from build123d import *

# Parameters (mm, degrees)
SKETCH2_R           = 12
BOSS_EXTRUDE1_DEPTH = 10.23
SKETCH3_R           = 2.5
CUT_EXTRUDE1_DEPTH  = 20.815471228
CHAMFER1_SIZE       = 2
CHAMFER2_SIZE       = 2


with BuildPart() as part:
    # Sketch2 → Boss-Extrude1 (new body)
    with BuildSketch(Plane.XY):
        Circle(SKETCH2_R)
    extrude(amount=BOSS_EXTRUDE1_DEPTH)

    # Sketch3 → Cut-Extrude1 (cut, through all)
    with BuildSketch(Plane.XY.offset(10.23)):
        Circle(SKETCH3_R)
    extrude(amount=-CUT_EXTRUDE1_DEPTH, mode=Mode.SUBTRACT)

    # Chamfer1
    chamfer1_edges = [part.edges().sort_by_distance(p)[0] for p in [
        (-12, 0, 10.23),
    ]]
    chamfer(chamfer1_edges, length=CHAMFER1_SIZE)

    # Chamfer2
    chamfer2_edges = [part.edges().sort_by_distance(p)[0] for p in [
        (-12, 0, 0),
    ]]
    chamfer(chamfer2_edges, length=CHAMFER2_SIZE)


solid = part.part
CAD build for the part. Positions are in the model's coordinates, mm. Give positions to 0.01 mm unless a question says otherwise; leave off trailing zeros. Order: outer loops, then holes, each group sorted by start corner. A loop starts at its lowest first (then second) coordinate and runs counter-clockwise, first axis right, second up. Notation, with made-up numbers: (38.5, 89.25) - (58.5, 89.25) arc R24 cw to (58.5, 112.25) - close; hole circle Ø9 at (60, 49.25). An arc over 180 degrees is marked (long way). Write each question's results on one line, items separated by ' | '.
1. Saw through at A-A on x = 0. List the corners of the cut face in (y, z), and give its area (3 significant figures).
Calculated:
outline: (-12, 2) - (-10, 0) - (-2.5, 0) - (-2.5, 10.23) - (-10, 10.23) - (-12, 8.23) - close; (2.5, 0) - (10, 0) - (12, 2) - (12, 8.23) - (10, 10.23) - (2.5, 10.23) - close | area: 186 mm2
2. Probe L1, parallel to Y at x = 0, z = 4.75; L2, parallel to Y at x = -0.5, z = 3.5; L3, parallel to X at y = 2, z = 7. List the from-to ranges inside material, lowest first. Write a range as from..to.
Calculated:
L1: y = -12..-2.5, 2.5..12 | L2: y = -11.99..-2.45, 2.45..11.99 | L3: x = -11.83..-1.5, 1.5..11.83
3. Pull direction Y, two halves, no side cores. Call faces 1 (the face through (2, -2, 10.23)), 2 (the face through (-0.54, -2.44, 5.19)), 3 (the face through (-11.99, 0.53, 5.07)): released by +Y, released by -Y, zero draft, split by the parting line, or undercut.
Calculated:
face 1: zero draft | face 2: undercut | face 3: split by the parting line
4. Saw through at C-C on z = 4. List the corners of the cut face in (x, y), and give its area (3 significant figures).
Calculated:
outline: circle Ø24 at (0, 0); hole circle Ø5 at (0, 0) | area: 433 mm2
5. Pin check, flat tip, straight feed: pin 1 (4 mm diameter, centred on x = 5, y = -7.5, fed in from -Z). Stop position of the tip, or through.
Calculated:
pin 1: stops at z = 0
